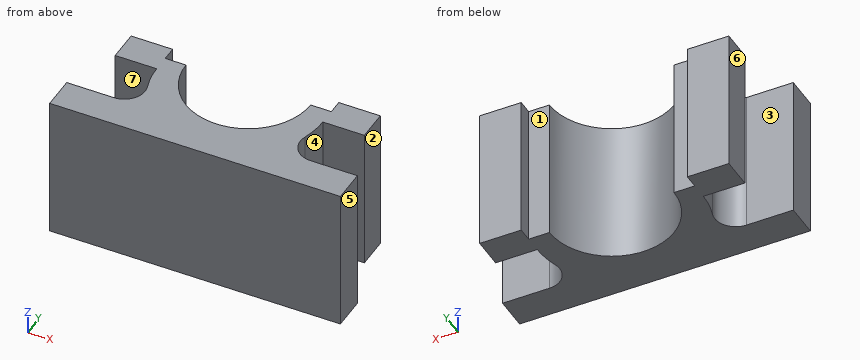
```python
from build123d import *

# Parameters (mm, degrees)
SALIENTE_EXTRUIR1_DEPTH = 105


with BuildPart() as part:
    # Croquis1 → Saliente-Extruir1 (new, symmetric)
    with BuildSketch(Plane.XY):
        with BuildLine():
            Line((-90, 0), (-120, 0))
            Line((-120, 0), (-120, 21))
            Line((-120, 21), (-180, 21))
            Line((-180, 21), (-180, -24))
            Line((-180, -24), (-120, -24))
            ThreePointArc((-120, -24), (-118.412019266, -43.457484251), (-113.69010511, -62.4))
            ThreePointArc((-113.69010511, -62.4), (-117.740516174, -89.492855685), (-142.112631388, -102))
            Line((-142.112631388, -102), (-210, -102))
            Line((-210, -102), (-210, -150))
            Line((-210, -150), (210, -150))
            Line((210, -150), (210, -102))
            Line((210, -102), (142.112631388, -102))
            ThreePointArc((142.112631388, -102), (117.740516174, -89.492855685), (113.69010511, -62.4))
            ThreePointArc((113.69010511, -62.4), (118.412019266, -43.457484251), (120, -24))
            Line((120, -24), (180, -24))
            Line((180, -24), (180, 21))
            Line((180, 21), (120, 21))
            Line((120, 21), (120, 0))
            Line((120, 0), (90, 0))
            ThreePointArc((90, 0), (0, -90), (-90, 0))
        make_face()
    extrude(amount=SALIENTE_EXTRUIR1_DEPTH, both=True)


solid = part.part
```
Build history of the part. All positions in model axes, mm. Face numbers are marked on the shaded views. A direction names the side the tool comes from. Give positions to 0.01 mm unless a question says otherwise; leave off trailing zeros. Order: outer loops, then holes, each group sorted by start corner. A loop starts at its lowest first (then second) coordinate and runs counter-clockwise, first axis right, second up. Notation, with made-up numbers: M -24,-1 L 26,-1 A11 ccw 26,3 Z; hole C 53,56.5 d5. An arc over 180 degrees is marked long. Return JSON: item names as keys, results as strings.
Q1. Band-saw the part on C-C (y = -68). Give the cut face in (x, z), then the cut area to 3 significant figures.
Answer list:
{"outline": "M -112.38,-105 L -58.96,-105 L -58.96,105 L -112.38,105 Z; M 58.96,-105 L 112.38,-105 L 112.38,105 L 58.96,105 Z", "area": "22,400 mm^2"}
Q2. Wall check: probe 1 along Y at (x, z) = (-124.5, -10.5); probe 2 along Y at (x, z) = (122, 40); probe 3 along X at (y, z) = (-71.5, 7). Give the ranges that are in metal, low to high. Write a range as from..to.
Answer list:
{"probe 1": "y = -150..-96.29, -24..21", "probe 2": "y = -150..-94.26, -24..21", "probe 3": "x = -112.12..-54.66, 54.66..112.12"}
Q3. Band-saw the part on B-B (z = 72.5). Give the cut face in (x, y).
Answer list:
{"outline": "M -210,-150 L 210,-150 L 210,-102 L 142.11,-102 A30 cw 113.69,-62.4 A120 ccw 120,-24 L 180,-24 L 180,21 L 120,21 L 120,0 L 90,0 A90 cw -90,0 L -120,0 L -120,21 L -180,21 L -180,-24 L -120,-24 A120 ccw -113.69,-62.4 A30 cw -142.11,-102 L -210,-102 Z"}
Q4. Band-saw the part on D-D (x = 0). Give the cut face in (y, z).
Answer list:
{"outline": "M -150,-105 L -90,-105 L -90,105 L -150,105 Z"}
Q5. Flat gauge pins, fed straight in: pin 1 (17 mm diameter, centred on y = 8.5, z = 39.5, fed in from +X); pin 2 (9 mm diameter, centred on x = 99, z = -6, fed in from +Y); pin 3 (10.5 mm diameter, centred on y = 7, z = -42.5, fed in from -X). Where does each tip first touch, or does it go through?
Answer list:
{"pin 1": "stops at x = 180", "pin 2": "stops at y = 0", "pin 3": "stops at x = -180"}
Q6. Two-plate mould, pull along X, no slides. Class the marked faces 1, 2 and 3: pulls with the +X half, pulls with the -X half, needs draft (parallel to the pull), parting line crosses it, or undercut.
Answer list:
{"face 1": "undercut", "face 2": "pulls with the +X half", "face 3": "needs draft"}
Q7. Band-saw the part on A-A (x = 155.5). Give the cut face in (y, z).
Answer list:
{"outline": "M -150,-105 L -102,-105 L -102,105 L -150,105 Z; M -24,-105 L 21,-105 L 21,105 L -24,105 Z"}
Q8. 3-axis set-ups, long thin cutter, end or side, ignore diameter. For the marked faces 4, 5, 6 and 7: which of +Z, -Z, +X, -X, +Y, -Y reach the whole face in a straight line?
Answer list:
{"face 4": "+Z, -Z, +X", "face 5": "+Z, -Z, +X, +Y, -Y", "face 6": "+Z, -Z, -X, +Y", "face 7": "+Z, -Z, -X"}
